The model under review builds one solid part; all positions refer to its coordinate system, in mm. Face numbers are marked on the shaded views. A direction names the side the tool comes from. Coordinates: 2 decimals unless noted, no trailing zeros. Loops run counter-clockwise (first coordinate to the right, second up) from the corner with the lowest first, then second, coordinate; pieces in that order, holes last. Notation, with made-up numbers: (15.5, 8.25) - (21.5, 8.25) arc R7 cw to (21.5, 17.25) - close; hole circle Ø5 at (59.25, 6.5). An arc over 180 degrees is marked (long way). Answer in a Markdown table with one row per item. Add a question column.
(1) Machinability: for the marked faces 5 and 6, which of the approach directions +Z, -Z, +X, -X, +Y, -Y give a long, thin tool a straight path to every point of the face, cutting with its end or side? Answer none if there is none.
(2) We need section A-A on y = 69. Write out the cut boundary in (x, z).
(3) We need section B-B on x = 63.5. Write out the cut boundary in (y, z), plus the area to 3 significant figures.
(4) For P1, Ø1.5, axis at x = -63.5, z = -62.5, coming from the +Y side, flat-tipped, find the tip position at first contact; note if it passes through.
(5) For line 1 along X through (y, z) = (142.5, 27); line 2 along Z through (x, y) = (98.5, 140), list the stretches that pass through material, from the lowest coordinate up.
(6) Mouldability with a two-part tool opening along Z and no side actions: class the marked faces 1, 2, 3 and 4 as +Z half, -Z half, draft (parallel to the pull), parting line (faces both ways), or undercut.
(7) We need section C-C on z = -27.5. Write out the cut boundary in (x, y), plus the area to 3 significant figures.
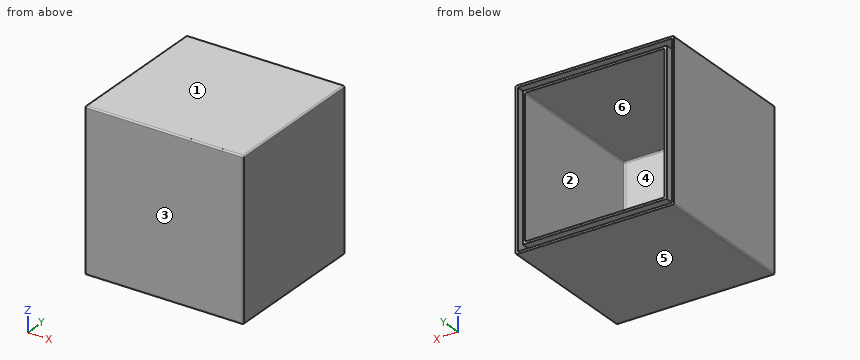
from build123d import *

# Parameters (mm, degrees)
SKETCH1_W             = 200
SKETCH1_H             = 200
SKETCH1_W_2           = 194
SKETCH1_H_2           = 194
BOSS_EXTRUDE1_DEPTH   = 205
SKETCH1_W_3           = 220
SKETCH1_H_3           = 220
SKETCH1_W_4           = 214
SKETCH1_H_4           = 214
BOSS_EXTRUDE1_2_DEPTH = 205
SKETCH3_W             = 220
SKETCH3_H             = 220
BOSS_EXTRUDE3_DEPTH   = 3
FILLET1_R             = 2


with BuildPart() as part:
    # Sketch1 → Boss-Extrude1 (new body)
    with BuildSketch(Plane(origin=(0, 0, 0), x_dir=(1, 0, 0), z_dir=(0, 1, 0))):
        Rectangle(SKETCH1_W, SKETCH1_H)
        Rectangle(SKETCH1_W_2, SKETCH1_H_2, mode=Mode.SUBTRACT)
    extrude(amount=BOSS_EXTRUDE1_DEPTH)



with BuildPart() as body_2:
    # Sketch1 → Boss-Extrude1 2 (new body)
    with BuildSketch(Plane(origin=(0, 0, 0), x_dir=(1, 0, 0), z_dir=(0, 1, 0))):
        Rectangle(SKETCH1_W_3, SKETCH1_H_3)
        Rectangle(SKETCH1_W_4, SKETCH1_H_4, mode=Mode.SUBTRACT)
    extrude(amount=BOSS_EXTRUDE1_2_DEPTH)


with BuildPart() as part_1:
    add(part.part)

    add(body_2.part)  # Boss-Extrude3 merges body 2
    # Sketch3 → Boss-Extrude3 (add)
    with BuildSketch(Plane.XZ):
        Rectangle(SKETCH3_W, SKETCH3_H)
    extrude(amount=BOSS_EXTRUDE3_DEPTH)

    # Fillet1
    fillet1_edges = [part_1.edges().sort_by_distance(p)[0] for p in [
        (-97, 0, 0),
        (0, 0, 97),
        (97, 0, 0),
        (0, 0, -97),
        (-97, 102.5, -97),
        (-97, 102.5, 97),
        (97, 102.5, 97),
        (97, 102.5, -97),
        (110, 101, -110),
        (110, 101, 110),
        (-110, 101, 110),
        (-110, 101, -110),
        (110, -3, 0),
        (0, -3, 110),
        (-110, -3, 0),
        (0, -3, -110),
    ]]
    fillet(fillet1_edges, radius=FILLET1_R)


solid = part_1.part
Outcome:
| question | item | result |
|---|---|---|
| 1 | face 5 | -Z, +X, -X, +Y, -Y |
| 1 | face 6 | +Y |
| 2 | outline | (-110, -108) arc R2 ccw to (-108, -110) - (108, -110) arc R2 ccw to (110, -108) - (110, 108) arc R2 ccw to (108, 110) - (-108, 110) arc R2 ccw to (-110, 108) - close; (-100, -100) - (100, -100) - (100, 100) - (-100, 100) - close; hole (-107, -107) - (107, -107) - (107, 107) - (-107, 107) - close; hole (-97, -95) arc R2 ccw to (-95, -97) - (95, -97) arc R2 ccw to (97, -95) - (97, 95) arc R2 ccw to (95, 97) - (-95, 97) arc R2 ccw to (-97, 95) - close |
| 3 | outline | (-3, -108) arc R2 ccw to (-1, -110) - (205, -110) - (205, -107) - (0, -107) - (0, -100) - (205, -100) - (205, -97) - (2, -97) arc R2 cw to (0, -95) - (0, 95) arc R2 cw to (2, 97) - (205, 97) - (205, 100) - (0, 100) - (0, 107) - (205, 107) - (205, 110) - (-1, 110) arc R2 ccw to (-3, 108) - close |
| 3 | area | 3,120 mm² |
| 4 | P1 | y = 0 |
| 5 | line 1 | -110 to -107, -100 to -97, 97 to 100, 107 to 110 |
| 5 | line 2 | -110 to -107, -100 to 100, 107 to 110 |
| 6 | face 1 | +Z half |
| 6 | face 2 | undercut |
| 6 | face 3 | draft |
| 6 | face 4 | undercut |
| 7 | outline | (-110, -1) arc R2 ccw to (-108, -3) - (108, -3) arc R2 ccw to (110, -1) - (110, 205) - (107, 205) - (107, 0) - (100, 0) - (100, 205) - (97, 205) - (97, 2) arc R2 cw to (95, 0) - (-95, 0) arc R2 cw to (-97, 2) - (-97, 205) - (-100, 205) - (-100, 0) - (-107, 0) - (-107, 205) - (-110, 205) - close |
| 7 | area | 3,120 mm² |
